from build123d import *

# Parameters (mm, degrees)
SKETCH1_W           = 131
SKETCH1_H           = 66
BOSS_EXTRUDE1_DEPTH = 1.5875
SKETCH3_W           = 117
SKETCH3_H           = 52
CUT_EXTRUDE2_DEPTH  = 74.360549045
SKETCH4_R           = 2
CUT_EXTRUDE3_DEPTH  = 74.360549045
FILLET1_R           = 3


with BuildPart() as part:
    # Sketch1 → Boss-Extrude1 (new body)
    with BuildSketch(Plane(origin=(0, 0, 0), x_dir=(1, 0, 0), z_dir=(0, 1, 0))):
        Rectangle(SKETCH1_W, SKETCH1_H)
    extrude(amount=BOSS_EXTRUDE1_DEPTH)

    # Sketch3 → Cut-Extrude2 (cut, through all)
    with BuildSketch(Plane(origin=(0, 1.5875, 0), x_dir=(1, 0, 0), z_dir=(0, 1, 0))):
        Rectangle(SKETCH3_W, SKETCH3_H)
    extrude(amount=-CUT_EXTRUDE2_DEPTH, mode=Mode.SUBTRACT)

    # Sketch4 → Cut-Extrude3 (cut, through all)
    with BuildSketch(Plane(origin=(0, 1.5875, 0), x_dir=(1, 0, 0), z_dir=(0, 1, 0))):
        with Locations(Location((-60.5, 28, 0), (0, 0, 270))):
            Circle(SKETCH4_R)
        with Locations(Location((60.5, 28, 0), (0, 0, 270))):
            Circle(SKETCH4_R)
        with Locations(Location((60.5, -28, 0), (0, 0, 270))):
            Circle(SKETCH4_R)
        with Locations(Location((-60.5, -28, 0), (0, 0, 270))):
            Circle(SKETCH4_R)
    extrude(amount=-CUT_EXTRUDE3_DEPTH, mode=Mode.SUBTRACT)

    # Fillet1
    fillet1_edges = [part.edges().sort_by_distance(p)[0] for p in [
        (-58.5, 0.79375, 26),
        (-58.5, 0.79375, -26),
        (58.5, 0.79375, -26),
        (58.5, 0.79375, 26),
        (-65.5, 0.79375, -33),
        (65.5, 0.79375, -33),
        (65.5, 0.79375, 33),
        (-65.5, 0.79375, 33),
    ]]
    fillet(fillet1_edges, radius=FILLET1_R)


solid = part.part
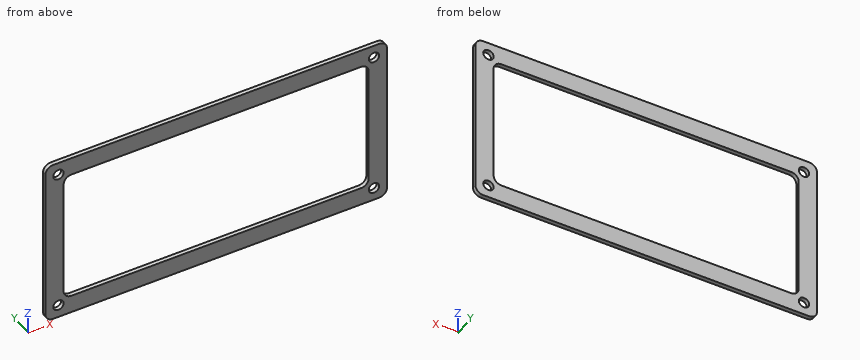
Could you check a few things on this model? Use its own coordinates, in mm. Round coordinates to 2 decimals unless told otherwise and drop trailing zeros. Loops run counter-clockwise (first coordinate to the right, second up) from the corner with the lowest first, then second, coordinate; pieces in that order, holes last. Notation, with made-up numbers: (2, 33.25) - (20, 33.25) arc R17 cw to (20, 63.25) - close; hole circle Ø3 at (85.25, 4). An arc over 180 degrees is marked (long way). Write item = value, one per line.
1) I need wall thicknesses on line 1 along X through (y, z) = (0.5, -28); line 2 along X through (y, z) = (1, -14.5); line 3 along Z through (x, y) = (-43.5, 1.2). Which ranges of each line are inside material? Lowest first, please. Write a range as from..to.
Computed:
line_1 = -65.5..-62.5, -58.5..58.5, 62.5..65.5
line_2 = -65.5..-58.5, 58.5..65.5
line_3 = -33..-26, 26..33
2) Imagine slicing it at B-B (x = 60.5). Please give me the cut outline in (y, z), and give its area (3 significant figures).
Computed:
outline = (0, -33) - (1.59, -33) - (1.59, -30) - (0, -30) - close; (0, -26) - (1.59, -26) - (1.59, 26) - (0, 26) - close; (0, 30) - (1.59, 30) - (1.59, 33) - (0, 33) - close
area = 92.1 mm2
3) I'm going to push flat-ended pins straight in: P1, Ø2.5, axis at x = -60.5, z = 28, coming from the +Y side; P2, Ø4.5, axis at x = 60.5, z = 28, coming from the +Y side. Where does each tip first touch, or does it pass through?
Computed:
P1 = through
P2 = 1.59
4) Imagine slicing it at C-C (z = -17.5). Please give me the cut outline in (x, y).
Computed:
outline = (-65.5, 0) - (-58.5, 0) - (-58.5, 1.59) - (-65.5, 1.59) - close; (58.5, 0) - (65.5, 0) - (65.5, 1.59) - (58.5, 1.59) - close
5) Imagine slicing it at A-A (z = 28). Please give me the cut outline in (x, y).
Computed:
outline = (-65.5, 0) - (-62.5, 0) - (-62.5, 1.59) - (-65.5, 1.59) - close; (-58.5, 0) - (58.5, 0) - (58.5, 1.59) - (-58.5, 1.59) - close; (62.5, 0) - (65.5, 0) - (65.5, 1.59) - (62.5, 1.59) - close
6) Imagine slicing it at D-D (x = -27). Please give me the cut outline in (y, z), and give its area (3 significant figures).
Computed:
outline = (0, -33) - (1.59, -33) - (1.59, -26) - (0, -26) - close; (0, 26) - (1.59, 26) - (1.59, 33) - (0, 33) - close
area = 22.2 mm2
